Source: CAD feature listing. Evaluate the final solid. Frame: model axes, mm. Give positions to 0.01 mm unless a question says otherwise; leave off trailing zeros. Order: outer loops, then holes, each group sorted by start corner. A loop starts at its lowest first (then second) coordinate and runs counter-clockwise, first axis right, second up. Notation, with made-up numbers: (-20, 19.5) -> (16, 19.5) arc R14 cw to (16, 33.5) -> close; hole circle Ø10 at (59, 27). An arc over 180 degrees is marked (long way). Answer in a Markdown table with one row per item.
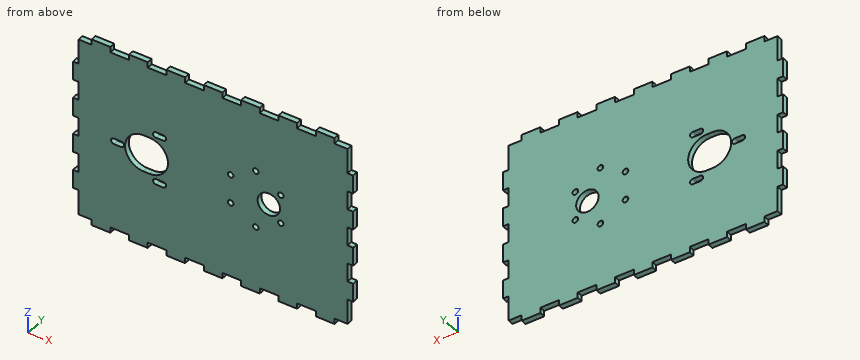
```python
from build123d import *

# Parameters (mm, degrees)
SKETCH1_W                 = 150
SKETCH1_H                 = 103
BOSS_EXTRUDE1_DEPTH       = 3
SKETCH2_W                 = 10
SKETCH2_H                 = 3
CUT_EXTRUDE1_DEPTH        = 92.028841583
LPATTERN1_COUNT           = 8
LPATTERN1_PITCH           = 20
MIRROR1_COPY_1_SKETCH_W   = 10
MIRROR1_COPY_1_SKETCH_H   = 3
MIRROR1_COPY_1_DEPTH      = 92.028841583
MIRROR1_COPY_2_SKETCH_W   = 10
MIRROR1_COPY_2_SKETCH_H   = 3
MIRROR1_COPY_2_DEPTH      = 92.028841583
MIRROR1_COPY_3_SKETCH_W   = 10
MIRROR1_COPY_3_SKETCH_H   = 3
MIRROR1_COPY_3_DEPTH      = 92.028841583
MIRROR1_COPY_4_SKETCH_W   = 10
MIRROR1_COPY_4_SKETCH_H   = 3
MIRROR1_COPY_4_DEPTH      = 92.028841583
MIRROR1_COPY_5_SKETCH_W   = 10
MIRROR1_COPY_5_SKETCH_H   = 3
MIRROR1_COPY_5_DEPTH      = 92.028841583
MIRROR1_COPY_6_SKETCH_W   = 10
MIRROR1_COPY_6_SKETCH_H   = 3
MIRROR1_COPY_6_DEPTH      = 92.028841583
MIRROR1_COPY_7_SKETCH_W   = 10
MIRROR1_COPY_7_SKETCH_H   = 3
MIRROR1_COPY_7_DEPTH      = 92.028841583
SKETCH3_W                 = 3
SKETCH3_H                 = 10
CUT_EXTRUDE2_DEPTH        = 92.028841583
LPATTERN2_COUNT           = 5
LPATTERN2_PITCH           = 20
MIRROR2_COPY_1_SKETCH_W   = 3
MIRROR2_COPY_1_SKETCH_H   = 10
MIRROR2_COPY_1_DEPTH      = 92.028841583
MIRROR2_COPY_2_SKETCH_W   = 3
MIRROR2_COPY_2_SKETCH_H   = 10
MIRROR2_COPY_2_DEPTH      = 92.028841583
MIRROR2_COPY_3_SKETCH_W   = 3
MIRROR2_COPY_3_SKETCH_H   = 10
MIRROR2_COPY_3_DEPTH      = 92.028841583
MIRROR2_COPY_4_SKETCH_W   = 3
MIRROR2_COPY_4_SKETCH_H   = 10
MIRROR2_COPY_4_DEPTH      = 92.028841583
SKETCH4_W                 = 3
SKETCH4_H                 = 3.5
CUT_EXTRUDE3_DEPTH        = 92.028841583
SKETCH7_R                 = 6
SKETCH7_R_2               = 1.5
CUT_EXTRUDE4_DEPTH        = 92.028841583
M3X0_5_TAPPED_HOLE3_D     = 3
M3X0_5_TAPPED_HOLE3_DEPTH = 10
M3X0_5_TAPPED_HOLE3_TIP   = 0.901290929


with BuildPart() as part:
    # Sketch1 → Boss-Extrude1 (new body)
    with BuildSketch(Plane(origin=(0, 0, 0), x_dir=(1, 0, 0), z_dir=(0, 1, 0))):
        Rectangle(SKETCH1_W, SKETCH1_H)
    extrude(amount=BOSS_EXTRUDE1_DEPTH)

    # Sketch2 → Cut-Extrude1 (cut, through all)
    with BuildSketch(Plane(origin=(0, 3, 0), x_dir=(1, 0, 0), z_dir=(0, 1, 0))):
        with Locations((70, -50)):
            Rectangle(SKETCH2_W, SKETCH2_H)
    cut_extrude1 = extrude(amount=-CUT_EXTRUDE1_DEPTH, mode=Mode.SUBTRACT)

    # LPattern1: Cut-Extrude1 ×8
    with Locations(*[(-i * LPATTERN1_PITCH, 0, 0) for i in range(1, LPATTERN1_COUNT)]):
        add(cut_extrude1, mode=Mode.SUBTRACT)

    # Mirror1: Cut-Extrude1 across plane
    add(cut_extrude1.mirror(Plane.XY), mode=Mode.SUBTRACT)

    # Mirror1 copy 1 sketch → Mirror1 copy 1 (cut, through all)
    with BuildSketch(Plane(origin=(-20, 3, 0), x_dir=(1, 0, 0), z_dir=(0, 1, 0))):
        with Locations((70, 50)):
            Rectangle(MIRROR1_COPY_1_SKETCH_W, MIRROR1_COPY_1_SKETCH_H)
    extrude(amount=-MIRROR1_COPY_1_DEPTH, mode=Mode.SUBTRACT)

    # Mirror1 copy 2 sketch → Mirror1 copy 2 (cut, through all)
    with BuildSketch(Plane(origin=(-40, 3, 0), x_dir=(1, 0, 0), z_dir=(0, 1, 0))):
        with Locations((70, 50)):
            Rectangle(MIRROR1_COPY_2_SKETCH_W, MIRROR1_COPY_2_SKETCH_H)
    extrude(amount=-MIRROR1_COPY_2_DEPTH, mode=Mode.SUBTRACT)

    # Mirror1 copy 3 sketch → Mirror1 copy 3 (cut, through all)
    with BuildSketch(Plane(origin=(-60, 3, 0), x_dir=(1, 0, 0), z_dir=(0, 1, 0))):
        with Locations((70, 50)):
            Rectangle(MIRROR1_COPY_3_SKETCH_W, MIRROR1_COPY_3_SKETCH_H)
    extrude(amount=-MIRROR1_COPY_3_DEPTH, mode=Mode.SUBTRACT)

    # Mirror1 copy 4 sketch → Mirror1 copy 4 (cut, through all)
    with BuildSketch(Plane(origin=(-80, 3, 0), x_dir=(1, 0, 0), z_dir=(0, 1, 0))):
        with Locations((70, 50)):
            Rectangle(MIRROR1_COPY_4_SKETCH_W, MIRROR1_COPY_4_SKETCH_H)
    extrude(amount=-MIRROR1_COPY_4_DEPTH, mode=Mode.SUBTRACT)

    # Mirror1 copy 5 sketch → Mirror1 copy 5 (cut, through all)
    with BuildSketch(Plane(origin=(-100, 3, 0), x_dir=(1, 0, 0), z_dir=(0, 1, 0))):
        with Locations((70, 50)):
            Rectangle(MIRROR1_COPY_5_SKETCH_W, MIRROR1_COPY_5_SKETCH_H)
    extrude(amount=-MIRROR1_COPY_5_DEPTH, mode=Mode.SUBTRACT)

    # Mirror1 copy 6 sketch → Mirror1 copy 6 (cut, through all)
    with BuildSketch(Plane(origin=(-120, 3, 0), x_dir=(1, 0, 0), z_dir=(0, 1, 0))):
        with Locations((70, 50)):
            Rectangle(MIRROR1_COPY_6_SKETCH_W, MIRROR1_COPY_6_SKETCH_H)
    extrude(amount=-MIRROR1_COPY_6_DEPTH, mode=Mode.SUBTRACT)

    # Mirror1 copy 7 sketch → Mirror1 copy 7 (cut, through all)
    with BuildSketch(Plane(origin=(-140, 3, 0), x_dir=(1, 0, 0), z_dir=(0, 1, 0))):
        with Locations((70, 50)):
            Rectangle(MIRROR1_COPY_7_SKETCH_W, MIRROR1_COPY_7_SKETCH_H)
    extrude(amount=-MIRROR1_COPY_7_DEPTH, mode=Mode.SUBTRACT)

    # Sketch3 → Cut-Extrude2 (cut, through all)
    with BuildSketch(Plane(origin=(0, 3, 0), x_dir=(1, 0, 0), z_dir=(0, 1, 0))):
        with Locations((73.5, 40)):
            Rectangle(SKETCH3_W, SKETCH3_H)
    cut_extrude2 = extrude(amount=-CUT_EXTRUDE2_DEPTH, mode=Mode.SUBTRACT)

    # LPattern2: Cut-Extrude2 ×5
    with Locations(*[(0, 0, i * LPATTERN2_PITCH) for i in range(1, LPATTERN2_COUNT)]):
        add(cut_extrude2, mode=Mode.SUBTRACT)

    # Mirror2: Cut-Extrude2 across plane
    add(cut_extrude2.mirror(Plane(origin=(0, 0, 0), x_dir=(0, 0, 1), z_dir=(1, 0, 0))), mode=Mode.SUBTRACT)

    # Mirror2 copy 1 sketch → Mirror2 copy 1 (cut, through all)
    with BuildSketch(Plane(origin=(0, 3, 20), x_dir=(-1, 0, 0), z_dir=(0, 1, 0))):
        with Locations((73.5, -40)):
            Rectangle(MIRROR2_COPY_1_SKETCH_W, MIRROR2_COPY_1_SKETCH_H)
    extrude(amount=-MIRROR2_COPY_1_DEPTH, mode=Mode.SUBTRACT)

    # Mirror2 copy 2 sketch → Mirror2 copy 2 (cut, through all)
    with BuildSketch(Plane(origin=(0, 3, 40), x_dir=(-1, 0, 0), z_dir=(0, 1, 0))):
        with Locations((73.5, -40)):
            Rectangle(MIRROR2_COPY_2_SKETCH_W, MIRROR2_COPY_2_SKETCH_H)
    extrude(amount=-MIRROR2_COPY_2_DEPTH, mode=Mode.SUBTRACT)

    # Mirror2 copy 3 sketch → Mirror2 copy 3 (cut, through all)
    with BuildSketch(Plane(origin=(0, 3, 60), x_dir=(-1, 0, 0), z_dir=(0, 1, 0))):
        with Locations((73.5, -40)):
            Rectangle(MIRROR2_COPY_3_SKETCH_W, MIRROR2_COPY_3_SKETCH_H)
    extrude(amount=-MIRROR2_COPY_3_DEPTH, mode=Mode.SUBTRACT)

    # Mirror2 copy 4 sketch → Mirror2 copy 4 (cut, through all)
    with BuildSketch(Plane(origin=(0, 3, 80), x_dir=(-1, 0, 0), z_dir=(0, 1, 0))):
        with Locations((73.5, -40)):
            Rectangle(MIRROR2_COPY_4_SKETCH_W, MIRROR2_COPY_4_SKETCH_H)
    extrude(amount=-MIRROR2_COPY_4_DEPTH, mode=Mode.SUBTRACT)

    # Sketch4 → Cut-Extrude3 (cut, through all)
    with BuildSketch(Plane(origin=(0, 3, 0), x_dir=(1, 0, 0), z_dir=(0, 1, 0))):
        with Locations((73.5, 46.75)):
            Rectangle(SKETCH4_W, SKETCH4_H)
        with Locations((-73.5, 46.75)):
            Rectangle(SKETCH4_W, SKETCH4_H)
        with Locations((-73.5, -46.75)):
            Rectangle(SKETCH4_W, SKETCH4_H)
        with Locations((73.5, -46.75)):
            Rectangle(SKETCH4_W, SKETCH4_H)
    extrude(amount=-CUT_EXTRUDE3_DEPTH, mode=Mode.SUBTRACT)

    # Sketch7 → Cut-Extrude4 (cut, through all)
    with BuildSketch(Plane(origin=(0, 3, 0), x_dir=(1, 0, 0), z_dir=(0, 1, 0))):
        with Locations(Location((29.848397993, 0, 0), (0, 0, 270))):
            Circle(SKETCH7_R)
        with Locations(Location((22.848397993, 15.5, 0), (0, 0, 270))):
            Circle(SKETCH7_R_2)
        with Locations(Location((36.271791752, 7.75, 0), (0, 0, 270))):
            Circle(SKETCH7_R_2)
        with Locations(Location((36.271791752, -7.75, 0), (0, 0, 270))):
            Circle(SKETCH7_R_2)
        with Locations(Location((22.848397993, -15.5, 0), (0, 0, 270))):
            Circle(SKETCH7_R_2)
        with Locations(Location((9.425004235, -7.75, 0), (0, 0, 270))):
            Circle(SKETCH7_R_2)
        with Locations(Location((9.425004235, 7.75, 0), (0, 0, 270))):
            Circle(SKETCH7_R_2)
        with BuildLine():
            Line((-34.151602007, -10), (-37.151602007, -10))
            ThreePointArc((-37.151602007, -10), (-47.151602007, 0), (-37.151602007, 10))
            Line((-37.151602007, 10), (-34.151602007, 10))
            ThreePointArc((-34.151602007, 10), (-24.151602007, 0), (-34.151602007, -10))
        make_face()
        with BuildLine():
            Line((-49.151602007, -1.5), (-53.151602007, -1.5))
            ThreePointArc((-53.151602007, -1.5), (-54.651602007, 0), (-53.151602007, 1.5))
            Line((-53.151602007, 1.5), (-49.151602007, 1.5))
            ThreePointArc((-49.151602007, 1.5), (-47.651602007, 0), (-49.151602007, -1.5))
        make_face()
        with BuildLine():
            Line((-26.651602007, 11.4685656), (-30.651602007, 11.4685656))
            ThreePointArc((-30.651602007, 11.4685656), (-32.151602007, 12.9685656), (-30.651602007, 14.4685656))
            Line((-30.651602007, 14.4685656), (-26.651602007, 14.4685656))
            ThreePointArc((-26.651602007, 14.4685656), (-25.151602007, 12.9685656), (-26.651602007, 11.4685656))
        make_face()
        with BuildLine():
            Line((-26.651602007, -14.512196514), (-30.651602007, -14.512196514))
            ThreePointArc((-30.651602007, -14.512196514), (-32.151602007, -13.012196514), (-30.651602007, -11.512196514))
            Line((-30.651602007, -11.512196514), (-26.651602007, -11.512196514))
            ThreePointArc((-26.651602007, -11.512196514), (-25.151602007, -13.012196514), (-26.651602007, -14.512196514))
        make_face()
    extrude(amount=-CUT_EXTRUDE4_DEPTH, mode=Mode.SUBTRACT)

    # M3x0.5 Tapped Hole3
    with Locations(Plane(origin=(0, 3, 0), x_dir=(1, 0, 0), z_dir=(0, 1, 0))):
        with Locations((22.848397993, 15.5), (36.271791752, -7.75), (22.848397993, -15.5), (9.425004235, -7.75), (9.425004235, 7.75), (36.271791752, 7.75)):
            Hole(M3X0_5_TAPPED_HOLE3_D / 2, depth=M3X0_5_TAPPED_HOLE3_DEPTH)
            with Locations((0, 0, -(M3X0_5_TAPPED_HOLE3_DEPTH + M3X0_5_TAPPED_HOLE3_TIP / 2))):  # 118° drill point
                Cone(0, M3X0_5_TAPPED_HOLE3_D / 2, M3X0_5_TAPPED_HOLE3_TIP, mode=Mode.SUBTRACT)


solid = part.part
```
(1) First-contact query: pin 1 Ø0.9 at (y, z) = (2, -50) entering from +X; pin 2 Ø1.5 at (y, z) = (1.5, -49.5) entering from -X; pin 3 Ø1.5 at (x, y) = (30.5, 1) entering from -Z. Flat tips, straight axial feed; report the tip coordinate or a pass-through.
A:
| item | result |
|---|---|
| pin 1 | stops at x = 65 |
| pin 2 | stops at x = -65 |
| pin 3 | stops at z = -48.5 |
(2) Section query A-A (z = 0). Return the cut outline in (x, y).
A:
| item | result |
|---|---|
| outline | (-72, 0) -> (-54.65, 0) -> (-54.65, 3) -> (-72, 3) -> close; (-47.65, 0) -> (-47.15, 0) -> (-47.15, 3) -> (-47.65, 3) -> close; (-24.15, 0) -> (23.85, 0) -> (23.85, 3) -> (-24.15, 3) -> close; (35.85, 0) -> (72, 0) -> (72, 3) -> (35.85, 3) -> close |
(3) Section query D-D (z = 19.5). Return the cut outline in (x, y), plus the area to 3 significant figures.
A:
| item | result |
|---|---|
| outline | (-72, 0) -> (72, 0) -> (72, 3) -> (-72, 3) -> close |
| area | 432 mm^2 |
(4) Ray query, probe 1 along X at (y, z) = (1.45, 0); probe 2 along X at (y, z) = (2.75, 13); probe 3 along Z at (x, y) = (-30.5, 1.05). Return the intervals inside material, ascending.
A:
| item | result |
|---|---|
| probe 1 | x = -72 to -54.65, -47.65 to -47.15, -24.15 to 23.85, 35.85 to 72 |
| probe 2 | x = -75 to -32.15, -25.15 to 75 |
| probe 3 | z = -48.5 to -14.47, -11.47 to -9.31, 9.31 to 11.51, 14.51 to 48.5 |
(5) Section query B-B (x = 49.5). Return the cut outline in (y, z), plus the area to 3 significant figures.
A:
| item | result |
|---|---|
| outline | (0, -48.5) -> (3, -48.5) -> (3, 48.5) -> (0, 48.5) -> close |
| area | 291 mm^2 |
(6) Section query C-C (y = 0.85). Give the number of separate pieces and of enclosed holes in the cut face, plus the area to 3 significant figures.
A:
| item | result |
|---|---|
| separate pieces | 1 |
| enclosed holes | 11 |
| area | 14,000 mm^2 |
